Part model, mm, in its own coordinate system. Round coordinates to 2 decimals unless told otherwise and drop trailing zeros. Write each loop counter-clockwise with the first axis right and the second up, starting at its lowest first coordinate (ties: lowest second). Pieces come first, ordered by that corner, then holes. Notation, with made-up numbers: (52, 64) -> (85, 64) arc R31 ccw to (85, 91) -> close; hole circle Ø6 at (-24.75, 17.5). An arc over 180 degrees is marked (long way). Use CSV: the item, a comma, the result in double quotes. Start each with the question number.
(1) Saw through at B-B (z = 0). Give the cut face in (x, y), plus the area to 3 significant figures.
(2) Probe line 1 (X direction, y = -3.6, z = 0); line 2 (X direction, y = 2.5, z = -5.5); line 3 (Z direction, x = 7, y = 1). List the from-to ranges inside material, lowest first. Write a range as [from, to].
(3) Saw through at A-A (x = 0). Give the cut face in (y, z).
(4) Saw through at C-C (y = 1). Give the cut face in (x, z).
(5) Drop flat-ended pins along their axis: pin 1 (1 mm diameter, centred on y = 2.5, z = 6.5, fed in from -X); pin 2 (3 mm diameter, centred on x = -4, y = 0.5, fed in from +Z); pin 3 (1.5 mm diameter, centred on x = 4.5, y = -2.5, fed in from -Z). Give the stop position or say it passes through.
```python
from build123d import *


with BuildPart() as part:
    # Sketch1 → Revolve1 (revolve)
    with BuildSketch(Plane.YZ, mode=Mode.PRIVATE) as revolve1_sk:
        with BuildLine():
            Line((-4, 17.5), (4, 17.5))
            ThreePointArc((4, 17.5), (4.707106781, 17.207106781), (5, 16.5))
            Line((5, 16.5), (5, 13.5))
            Line((5, 13.5), (2.291287847, 13.5))
            ThreePointArc((2.291287847, 13.5), (0, 15), (-2.291287847, 13.5))
            Line((-2.291287847, 13.5), (-5, 13.5))
            Line((-5, 13.5), (-5, 16.5))
            ThreePointArc((-5, 16.5), (-4.707106781, 17.207106781), (-4, 17.5))
        make_face()
    revolve(revolve1_sk.sketch.rotate(Axis((0, -30.435284328, 0), (0, 1, 0)), 180), axis=Axis((0, -30.435284328, 0), (0, 1, 0)))


solid = part.part
```
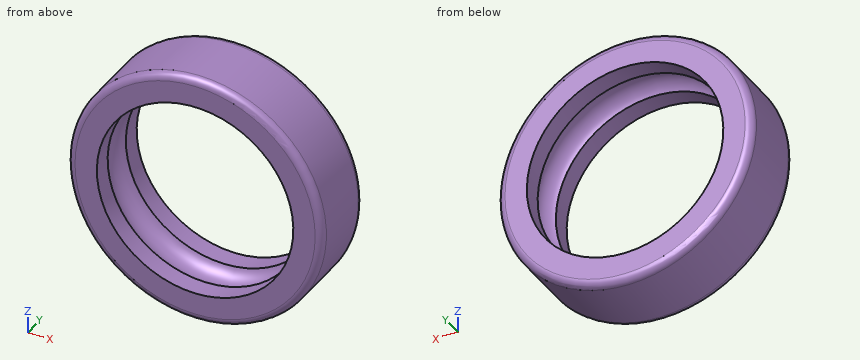
Answers:
1,outline,"(-17.5, -4) arc R1 ccw to (-16.5, -5) -> (-13.5, -5) -> (-13.5, -2.29) arc R2.5 cw to (-13.5, 2.29) -> (-13.5, 5) -> (-16.5, 5) arc R1 ccw to (-17.5, 4) -> close; (13.5, -5) -> (16.5, -5) arc R1 ccw to (17.5, -4) -> (17.5, 4) arc R1 ccw to (16.5, 5) -> (13.5, 5) -> (13.5, 2.29) arc R2.5 cw to (13.5, -2.29) -> close"
1,area,"69.2 mm²"
2,line 1,"x = [-17.5, -13.5], [13.5, 17.5]"
2,line 2,"x = [-16.61, -12.33], [12.33, 16.61]"
2,line 3,"z = [-16.04, -13.03], [13.03, 16.04]"
3,outline,"(-5, -16.5) arc R1 ccw to (-4, -17.5) -> (4, -17.5) arc R1 ccw to (5, -16.5) -> (5, -13.5) -> (2.29, -13.5) arc R2.5 cw to (-2.29, -13.5) -> (-5, -13.5) -> close; (-5, 13.5) -> (-2.29, 13.5) arc R2.5 cw to (2.29, 13.5) -> (5, 13.5) -> (5, 16.5) arc R1 ccw to (4, 17.5) -> (-4, 17.5) arc R1 ccw to (-5, 16.5) -> close"
4,outline,"circle Ø35 at (0, 0); hole circle Ø29.58 at (0, 0)"
5,pin 1,"stops at x = -16.44"
5,pin 2,"stops at z = 17.32"
5,pin 3,"stops at z = -17.09"
